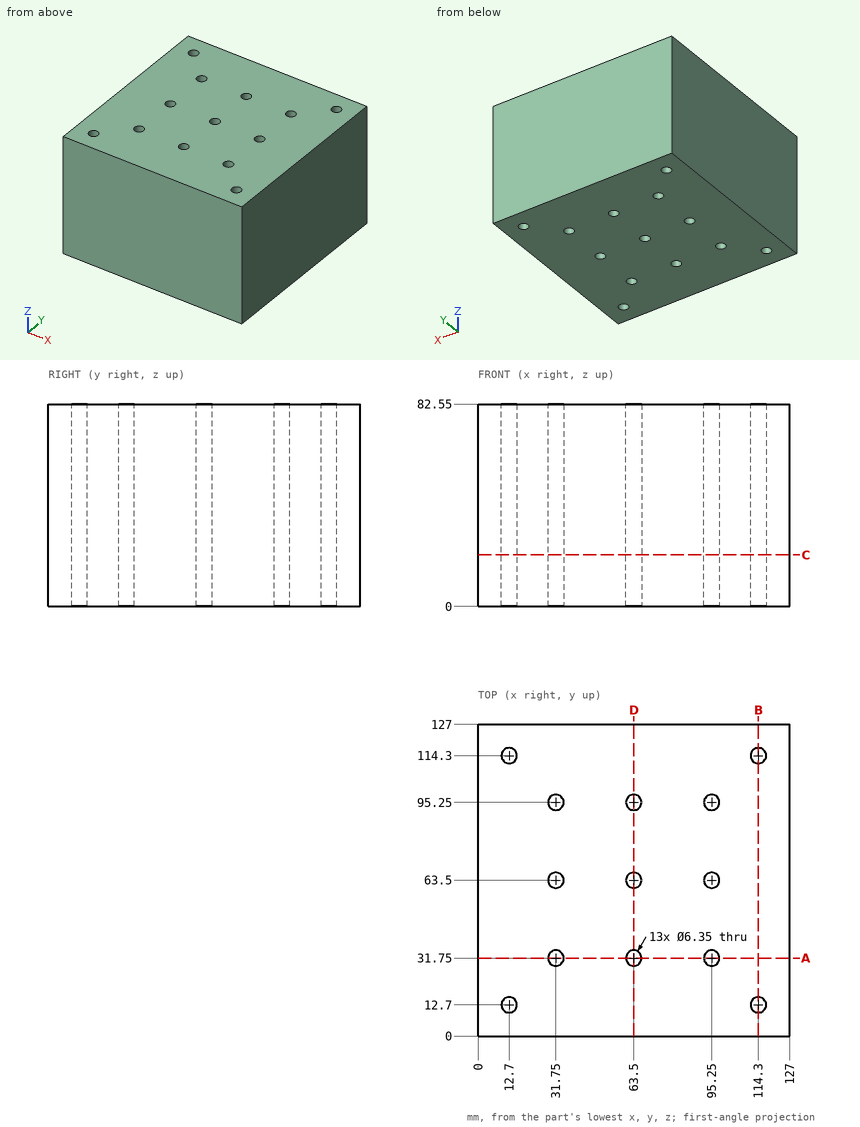
Drawing for the job (mm, zero at the part's lowest x, y, z). Coordinates: 2 decimals unless noted, no trailing zeros. Order: outer loops, then holes, each group sorted by start corner. A loop starts at its lowest first (then second) coordinate and runs counter-clockwise, first axis right, second up. Notation, with made-up numbers: (30.25, 50.5) -> (63.25, 50.5) arc R8 cw to (63.25, 64.5) -> close; hole circle Ø3 at (43, -3.75). An arc over 180 degrees is marked (long way). Return JSON: item names as keys, results as strings.
Item 1: Slice it at A-A (y = 31.75). Write the cut outline in (x, z) (3 decimals), then the cut area to 3 significant figures.
Model answer:
{"outline": "(0, 0) -> (28.575, 0) -> (28.575, 82.55) -> (0, 82.55) -> close; (34.925, 0) -> (60.325, 0) -> (60.325, 82.55) -> (34.925, 82.55) -> close; (66.675, 0) -> (92.075, 0) -> (92.075, 82.55) -> (66.675, 82.55) -> close; (98.425, 0) -> (127, 0) -> (127, 82.55) -> (98.425, 82.55) -> close", "area": "8,910 mm²"}
Item 2: Slice it at C-C (z = 21). Count the separate pieces of the cut face and the enclosed holes in it, then the cut area to 3 significant figures.
Model answer:
{"separate pieces": "1", "enclosed holes": "13", "area": "15,700 mm²"}
Item 3: Slice it at B-B (x = 114.3). Write the cut outline in (y, z) (3 decimals).
Model answer:
{"outline": "(0, 0) -> (9.525, 0) -> (9.525, 82.55) -> (0, 82.55) -> close; (15.875, 0) -> (111.125, 0) -> (111.125, 82.55) -> (15.875, 82.55) -> close; (117.475, 0) -> (127, 0) -> (127, 82.55) -> (117.475, 82.55) -> close"}
Item 4: Wall check: line 1 along Y through (x, z) = (32, 27); line 2 along Y through (x, z) = (12.7, 61.5) (3 decimals); line 3 along X through (y, z) = (63, 18). Give the ranges that are in metal, low to high. Write a range as from..to.
Model answer:
{"line 1": "y = 0..28.58, 34.92..60.33, 66.67..92.08, 98.42..127", "line 2": "y = 0..9.525, 15.875..111.125, 117.475..127", "line 3": "x = 0..28.61, 34.89..60.36, 66.64..92.11, 98.39..127"}
